Work out the finished part from the listing and answer in its coordinate system (mm). Face numbers are marked on the shaded views. A direction names the side the tool comes from. Coordinates: 2 decimals unless noted, no trailing zeros. Order: outer loops, then holes, each group sorted by start corner. A loop starts at its lowest first (then second) coordinate and runs counter-clockwise, first axis right, second up. Notation, with made-up numbers: (26, 84) -> (42, 84) arc R29 cw to (42, 117) -> close; hole circle Ø4 at (78.25, -1). An arc over 180 degrees is marked (long way). Write item = value, one per line. Start each with the question number.
Q1. For a pull along Z with two mould halves and no side action, classify the marked faces 5, 6 and 7 as +Z half, -Z half, draft (parallel to the pull), parting line (faces both ways), or undercut.
Q2. Which of the six approach directions +Z, -Z, +X, -X, +Y, -Y give full straight-line access (tool end or side, diameter ignored) to the marked faces 1, 2, 3 and 4?
Q3. Flat-ended cylindrical pins translate along their axes: pin 1 (2 mm diameter, centred on y = 60, z = -5, fed in from -X); pin 2 (1.3 mm diameter, centred on y = 59.5, z = -5, fed in from +X); pin 3 (1 mm diameter, centred on y = 13, z = 23, fed in from +X). Find the tip coordinate at first contact, or state that the pin passes through.
Q4. The part is cut by section B-B, the plane x = 0. Determine the outline of the cut face in (y, z), plus the area to 3 significant figures.
Q5. The part is cut by section A-A, the plane z = 0. Determine the outline of the cut face in (x, y).
Q6. Straight lines are drawn through the part: L1, parallel to Z at x = 0, y = 2.5; L2, parallel to Y at x = 10.8, z = 5; L3, parallel to Z at x = 10, y = 60. For each, find the intervals that lie inside material, in ascending order. Write a range as from..to.
Q7. The part is cut by section C-C, the plane y = 29. Determine the outline of the cut face in (x, z).
Q8. The part is cut by section D-D, the plane y = 50. Determine the outline of the cut face in (x, z), plus the area to 3 significant figures.
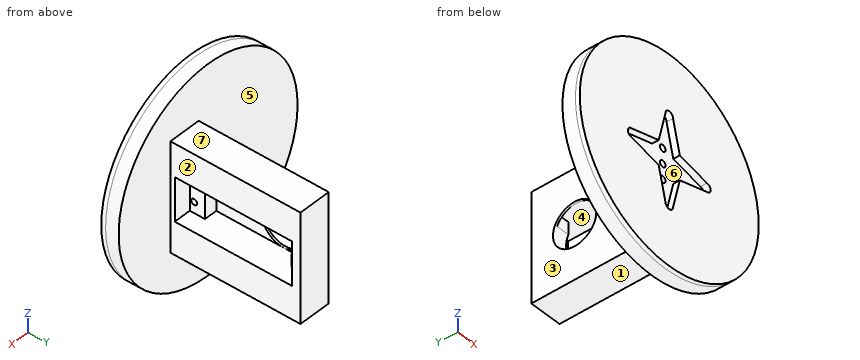
Autodesk Inventor part; units mm, degrees
ref_plane "YZ Plane" through (0, 0, 0) normal (1, 0, 0) x (0, 1, 0)
ref_plane "XZ Plane" through (0, 0, 0) normal (0, 1, 0) x (-1, 0, 0)
ref_plane "XY Plane" through (0, 0, 0) normal (0, 0, 1) x (1, 0, 0)
sketch "Sketch1" plane through (0, 0, 0) normal (0, 1, 0) x (-1, 0, 0)
  circle A0 centre (0, 0) radius 47.5
  dimension "d0" = 95
extrude "Extrusion1" add sketch "Sketch1" along normal blind 6
sketch "Sketch2" plane through (0, 6, 0) normal (0, 1, 0) x (1, 0, 0)
  circle A0 centre (0, 0) radius 7
  circle A1 centre (0, -7) radius 1.5
  circle A2 centre (0, 7) radius 1.5
  dimension "d3" = 14
  dimension "d4" = 3
  dimension "d5" = 3
extrude "Extrusion2" cut sketch "Sketch2" against normal blind 6 contours A2 A0 | A0 A2 | A1 A0 | A0 A1
sketch "Sketch3" plane through (0, 6, 0) normal (0, 1, 0) x (1, 0, 0)
  line L0 (0, 0) -> (5, 0)
  line L1 (5, 0) -> (5, -10)
  line L2 (5, -10) -> (0, -10)
  line L3 (0, -10) -> (0, 0)
  line L4 (5, 0) -> (0, 0)
  line L5 (0, 0) -> (0, 10)
  line L6 (0, 10) -> (5, 10)
  line L7 (5, 10) -> (5, 0)
  line L8 (5, 0) -> (20, 0)
  line L9 (20, 0) -> (20, -25)
  line L10 (20, -25) -> (5, -25)
  line L11 (5, -25) -> (5, 0)
  line L12 (20, 0) -> (5, 0)
  line L13 (5, 0) -> (5, 25)
  line L14 (5, 25) -> (20, 25)
  line L15 (20, 25) -> (20, 0)
  dimension "d8" = 5
  dimension "d9" = 10
  dimension "d10" = 10
  dimension "d11" = 15
  dimension "d12" = 25
  dimension "d13" = 25
extrude "Extrusion3" add sketch "Sketch3" along normal blind 60 contours L8 L9 L10 L11 L1 | L7 L13 L14 L15 L8
sketch "Sketch4" plane through (5, 6, -25) normal (-1, 0, 0) x (0, 0, 1)
  line L0 (50, 0) -> (50, 60)
  line L1 (50, 0) -> (48, 0)
  line L2 (48, 0) -> (48, 40)
  line L3 (48, 40) -> (50, 40)
  line L4 (50, 40) -> (50, 0)
  circle A0 centre (25, 40) radius 10
  point P0 (25, -6)
  dimension "d16" = 2
  dimension "d17" = 40
  dimension "d18" = 20
extrude "Extrusion4" cut sketch "Sketch4" against normal blind 20 contours A0
sketch "Sketch5" plane through (20, 6, 25) normal (1, 0, 0) x (0, 0, -1)
  circle A0 centre (25, 40) radius 10
  line L0 (25, 40) -> (30, 40)
  line L1 (30, 40) -> (30, 4)
  line L2 (30, 4) -> (25, 4)
  line L3 (25, 4) -> (25, 40)
  line L4 (25, 40) -> (20, 40)
  line L5 (20, 40) -> (20, 4)
  line L6 (20, 4) -> (25, 4)
  line L7 (25, 4) -> (25, 40)
  circle A1 centre (20, 4) radius 1.35
  circle A2 centre (30, 4) radius 1.35
  point P0 (25, -6)
  dimension "d21" = 5
  dimension "d22" = 36
  dimension "d23" = 5
  dimension "d24" = 36
  dimension "d25" = 2.7
  dimension "d26" = 2.7
extrude "Extrusion5" cut sketch "Sketch5" against normal blind 20 contours A1 L6 L5 | L5 L6 A1 | A2 L2 L1 | L1 L2 A2
sketch "Sketch6" plane through (20, 6, 25) normal (1, 0, 0) x (0, 0, -1)
  line L0 (25, 40) -> (30, 40)
  line L1 (30, 40) -> (30, 54)
  line L2 (30, 54) -> (25, 54)
  line L3 (25, 54) -> (25, 40)
  line L4 (25, 40) -> (20, 40)
  line L5 (20, 40) -> (20, 54)
  line L6 (20, 54) -> (25, 54)
  line L7 (25, 54) -> (25, 40)
  circle A0 centre (20, 54) radius 1.35
  circle A1 centre (30, 54) radius 1.35
  point P0 (25, -6)
  dimension "d29" = 5
  dimension "d30" = 14
  dimension "d31" = 5
  dimension "d32" = 14
  dimension "d33" = 2.7
  dimension "d34" = 2.7
extrude "Extrusion6" cut sketch "Sketch6" against normal blind 20 contours A1 L2 L1 | L1 L2 A1 | A0 L5 L6 | L6 L5 A0
sketch "Sketch7" plane through (20, 6, 25) normal (1, 0, 0) x (0, 0, -1)
  line L0 (20, 54) -> (30, 54)
  line L1 (30, 54) -> (30, 4)
  line L2 (30, 4) -> (20, 4)
  line L3 (20, 4) -> (20, 54)
  circle A0 centre (20, 54) radius 1.35
  line L4 (0, 0) -> (0, 60)
  line L5 (20, 54) -> (0, 54)
  line L6 (0, 54) -> (0, 49)
  line L7 (0, 49) -> (20, 49)
  line L8 (20, 49) -> (20, 54)
  circle A1 centre (25, 40) radius 10
  line L9 (25, 40) -> (15, 40)
  line L10 (15, 40) -> (15, 30)
  line L11 (15, 30) -> (25, 30)
  line L12 (25, 30) -> (25, 40)
  line L13 (25, 40) -> (35, 40)
  line L14 (35, 40) -> (35, 30)
  line L15 (35, 30) -> (25, 30)
  line L16 (25, 30) -> (25, 40)
  line L17 (35, 40) -> (15, 40)
  line L18 (15, 40) -> (15, 9)
  line L19 (15, 9) -> (35, 9)
  line L20 (35, 9) -> (35, 40)
  line L21 (15, 9) -> (35, 9)
  line L22 (35, 9) -> (35, 49)
  line L23 (35, 49) -> (15, 49)
  line L24 (15, 49) -> (15, 9)
  point P0 (25, -6)
  point P1 (30, 49)
  point P2 (30, 48.6603)
  point P3 (15, 49)
  point P4 (20, 48.6603)
  dimension "d37" = 10
  dimension "d38" = 50
  dimension "d39" = 5
  dimension "d40" = 10
  dimension "d41" = 10
  dimension "d42" = 10
  dimension "d43" = 31
  dimension "d44" = 40
extrude "Extrusion7" cut sketch "Sketch7" against normal blind 14 contours L3 A1 L24 L7 | L23 L22 A1 L1 | A1 L3 L11 L10 | L14 L15 L1 A1 | A1 L11 L3 | L11 L3 L19 L18 | L1 L15 A1 | L20 L19 L1 L15 | L11 L15 L1 L19 L3
sketch "Sketch8" plane through (20, 6, 25) normal (1, 0, 0) x (0, 0, -1)
  line L0 (15, 40) -> (15, 49)
  line L1 (15, 49) -> (35, 49)
  line L2 (35, 49) -> (35, 56)
  line L3 (35, 56) -> (15, 56)
  line L4 (15, 56) -> (15, 49)
  line L5 (35, 9) -> (15, 9)
  line L6 (15, 9) -> (35, 9)
  line L7 (35, 9) -> (35, 2)
  line L8 (35, 2) -> (15, 2)
  line L9 (15, 2) -> (15, 9)
  point P0 (25, -6)
  dimension "d47" = 20
  dimension "d48" = 7
  dimension "d49" = 20
  dimension "d50" = 7
sketch "Sketch9" plane through (20, 6, 25) normal (1, 0, 0) x (0, 0, -1)
  line L0 (15, 40) -> (15, 49)
  circle A0 centre (25, 40) radius 10
  line L1 (15, 49) -> (35, 49)
  line L2 (35, 49) -> (35, 40)
  line L3 (35, 40) -> (15, 40)
  line L4 (15, 40) -> (15, 49)
  line L5 (15, 49) -> (20, 49)
  line L6 (20, 49) -> (20.777, 49)
  line L7 (20.777, 49) -> (20.777, 48.469)
  line L8 (20.777, 48.469) -> (20, 48.469)
  line L9 (20, 48.469) -> (20, 49)
  line L10 (30, 49) -> (35, 49)
  line L11 (30, 49) -> (29.2041, 49)
  line L12 (29.2041, 49) -> (29.2041, 48.469)
  line L13 (29.2041, 48.469) -> (30, 48.469)
  line L14 (30, 48.469) -> (30, 49)
  line L15 (35, 49) -> (35, 9)
  line L16 (15, 56) -> (35, 56)
  line L17 (35, 56) -> (35, 49)
  line L18 (35, 49) -> (15, 49)
  line L19 (15, 49) -> (15, 56)
  line L20 (15, 9) -> (15, 49)
  line L21 (15, 9) -> (35, 9)
  line L22 (35, 9) -> (35, 2)
  line L23 (35, 2) -> (15, 2)
  line L24 (15, 2) -> (15, 9)
  point P0 (25, -6)
  point P1 (20, 48.6603)
  point P2 (30, 48.6603)
  dimension "d51" = 7
extrude "Extrusion8" cut sketch "Sketch9" against normal blind 12 contours L19 L16 L17 L1 A0 | L9 L1 A0 | L21 L22 L23 L24 | A0 L1 L14
sketch "Sketch10" plane through (8, 60, -5) normal (1, 0, 0) x (0, 0, -1)
  line L0 (-10, -5) -> (-10, -5.3397)
  line L1 (-10, -5) -> (0, -5)
  line L2 (0, -5) -> (0, -5.5581)
  line L3 (0, -5.5581) -> (-10, -5.5581)
  line L4 (-10, -5.5581) -> (-10, -5)
  point P0 (-5, -60)
extrude "Extrusion9" cut sketch "Sketch10" against normal blind 2
sketch "Sketch11" plane through (5, 6, -25) normal (-1, 0, 0) x (0, 0, 1)
  point P0 (25, -6)
sketch "Sketch12" plane through (0, 0, 0) normal (0, -1, 0) x (1, 0, 0)
  circle A0 centre (0, 0) radius 1.5
  dimension "d56" = 3
extrude "Extrusion10" cut sketch "Sketch12" against normal blind 13.8125
sketch "Sketch13" plane through (0, 0, 0) normal (0, -1, 0) x (1, 0, 0)
  circle A0 centre (0, 0) radius 1.5
  circle A1 centre (0, 0) radius 47.5
  circle A2 centre (0, 7) radius 1.5
  circle A3 centre (0, 7) radius 1.5
  circle A4 centre (0, 0) radius 1.5
  circle A5 centre (0, -7) radius 1.5
  circle A6 centre (0, -7) radius 1.5
  dimension "d59" = 3
extrude "Extrusion11" add sketch "Sketch13" along normal blind 2
sketch "Sketch14" plane through (0, -2, 0) normal (0, -1, 0) x (1, 0, 0)
  circle A0 centre (0, 0) radius 1.5
  circle A1 centre (0, 0) radius 7
  line L0 (0, 0) -> (0, -20)
  line L1 (0, -20) -> (0, 20)
  line L2 (0, 0) -> (20, 0)
  line L3 (20, 0) -> (-20, 0)
  circle A2 centre (0, 20) radius 2
  circle A3 centre (-20, 0) radius 2
  circle A4 centre (0, -20) radius 2
  circle A5 centre (20, 0) radius 2
  line L4 (2, 20) -> (7, 0)
  line L5 (-2, 20) -> (-7, 0)
  line L6 (20, 25) -> (20, -25)
  circle A6 centre (0, 7) radius 1.5
  line L7 (20, 2) -> (0, 7)
  circle A7 centre (0, -7) radius 1.5
  line L8 (20, -2) -> (0, -7)
  line L9 (2, -20) -> (7, 0)
  line L10 (-2, -20) -> (-7, 0)
  line L11 (-20, 2) -> (0, 7)
  line L12 (-20, -2) -> (0, -7)
  point P0 (6.1765, 3.2941)
  point P1 (6.1765, -3.2941)
  point P2 (-6.1765, -3.2941)
  point P3 (3.2941, -6.1765)
  point P4 (1.4914, -6.8393)
  point P5 (-1.4914, -6.8393)
  point P6 (-3.2941, -6.1765)
  point P7 (-1.4552, -6.6362)
  point P8 (1.4552, -6.6362)
  point P9 (3.2941, 6.1765)
  point P10 (1.4552, 6.6362)
  point P11 (-1.4552, 6.6362)
  point P12 (-3.2941, 6.1765)
  point P13 (-1.4914, 6.8393)
  point P14 (1.4914, 6.8393)
  point P15 (5.6, 5.6)
  point P16 (-5.6, 5.6)
  point P17 (-5.6, -5.6)
  point P18 (5.6, -5.6)
  dimension "d62" = 14
  dimension "d63" = 20
  dimension "d64" = 40
  dimension "d65" = 20
  dimension "d66" = 40
  dimension "d67" = 4
  dimension "d68" = 4
  dimension "d69" = 4
  dimension "d70" = 4
extrude "Extrusion12" cut sketch "Sketch14" against normal blind 3 contours L2 L9 A1 L8 A7 L0 A0 | A0 L1 A6 L7 A1 L4 L2 | A0 L3 L5 A1 L11 A6 L1 | L0 A7 L12 A1 L10 L3 A0 | L2 A5 L8 L9 A1 | A1 L4 L7 A5 L2 | A1 L7 L4 | L9 L8 A1 | A5 L6 L2 | L2 L6 A5 | L3 A3 L11 L5 A1 | A1 L10 L12 A3 L3 | A1 L5 | A1 A6 L1 A2 L4 L7 | L8 L9 A4 L0 A7 A1 | L6 A5 | L5 L11 A1 | A1 L12 L10 | A3 | A1 L11 L5 A2 L1 A6 | A7 L0 A4 L10 L12 A1 | A2 | A4
sketch "Sketch16" plane through (0, -2, 0) normal (0, -1, 0) x (1, 0, 0)
  line L0 (-8.315, -3.9346) -> (-4.5008, -3.9346)
  line L1 (-4.5008, -3.9346) -> (-4.5008, 0)
  line L2 (-4.5008, 0) -> (-8.315, 0)
  line L3 (-8.315, 0) -> (-8.315, -3.9346)
  line L4 (-3.8, -5.15) -> (4.3559, -5.15)
  line L5 (4.3559, -5.15) -> (4.3559, -8.3953)
  line L6 (4.3559, -8.3953) -> (-3.8, -8.3953)
  line L7 (-3.8, -8.3953) -> (-3.8, -5.15)
  line L8 (-3.8, 4.0171) -> (3.8, 4.0171)
  line L9 (3.8, 4.0171) -> (3.8, 8.6071)
  line L10 (3.8, 8.6071) -> (-3.8, 8.6071)
  line L11 (-3.8, 8.6071) -> (-3.8, 4.0171)
  line L12 (6, -4.3589) -> (8, -4.3589)
  line L13 (5.3903, 4.0171) -> (8, 4.0171)
  line L14 (8, 4.0171) -> (8, -4.3589)
  line L15 (8, -4.3589) -> (5.3903, -4.3589)
  line L16 (5.3903, -4.3589) -> (5.3903, 4.0171)
  point P0 (0, 0)
extrude "Extrusion13" cut sketch "Sketch16" against normal blind 3
sketch "Sketch17" plane through (8, 6, 25) normal (1, 0, 0) x (0, 0, -1)
  point P0 (25, -6)
sketch "Sketch18" plane through (6, 15, 10) normal (0, 0, -1) x (-1, 0, 0)
  point P0 (6, -15)
sketch "Sketch19" plane through (6, 15, 10) normal (0, 1, 0) x (1, 0, 0)
  point P0 (-6, 10)
sketch "Sketch20" plane through (8, 6, 25) normal (1, 0, 0) x (0, 0, -1)
  line L0 (35, 56) -> (35, 2)
  line L1 (15, 49) -> (20.6411, 49)
  line L2 (35, 56) -> (15, 56)
  line L3 (15, 56) -> (15, 49)
  line L4 (15, 49) -> (35, 49)
  line L5 (35, 49) -> (35, 56)
  circle A0 centre (25, 40) radius 10
  circle A1 centre (25, 40) radius 10
  line L6 (35, 40) -> (35, 9)
  line L7 (35, 2) -> (15, 2)
  line L8 (35, 9) -> (15, 9)
  line L9 (15, 9) -> (15, 2)
  line L10 (15, 2) -> (35, 2)
  line L11 (35, 2) -> (35, 9)
  circle A2 centre (20, 54) radius 1.35
  circle A3 centre (20, 54) radius 0.875
  circle A4 centre (30, 54) radius 1.35
  circle A5 centre (30, 54) radius 0.875
  circle A6 centre (30, 4) radius 1.35
  circle A7 centre (30, 4) radius 0.875
  circle A8 centre (20, 4) radius 1.35
  circle A9 centre (20, 4) radius 0.875
  point P0 (25, -6)
  point P1 (29.3589, 49)
extrude "Extrusion14" add sketch "Sketch20" along normal blind 8 contours L0 L7 L9 L8 | L0 L4 A0 L1 L3 L2
sketch "Sketch21" plane through (5, 6, -25) normal (-1, 0, 0) x (0, 0, 1)
  circle A0 centre (30, 54) radius 1.35
  circle A1 centre (30, 54) radius 1.35
  circle A2 centre (20, 54) radius 1.35
  circle A3 centre (20, 54) radius 1.35
  circle A4 centre (30, 4) radius 1.35
  circle A5 centre (30, 4) radius 1.35
  circle A6 centre (20, 4) radius 1.35
  circle A7 centre (20, 4) radius 1.35
  point P0 (25, -6)
extrude "Extrusion15" add sketch "Sketch21" against normal blind 2
sketch "Sketch22" plane through (16, 6, 25) normal (1, 0, 0) x (0, 0, -1)
  line L0 (15, 56) -> (35, 56)
  line L1 (15, 49) -> (15, 56)
  line L2 (35, 56) -> (15, 56)
  line L3 (15, 56) -> (15, 49)
  line L4 (15, 49) -> (35, 49)
  line L5 (35, 49) -> (35, 56)
  arc A0 (35, 40) -> (29.3589, 49) centre (25, 40) ccw
  circle A1 centre (25, 40) radius 10
  line L6 (35, 9) -> (15, 9)
  line L7 (35, 2) -> (15, 2)
  line L8 (15, 9) -> (35, 9)
  line L9 (35, 9) -> (35, 2)
  line L10 (35, 2) -> (15, 2)
  line L11 (15, 2) -> (15, 9)
  circle A2 centre (30, 54) radius 1.35
  circle A3 centre (30, 54) radius 1.35
  circle A4 centre (20, 54) radius 1.35
  circle A5 centre (20, 54) radius 1.35
  circle A6 centre (30, 4) radius 1.35
  circle A7 centre (30, 4) radius 1.35
  circle A8 centre (20, 4) radius 1.35
  circle A9 centre (20, 4) radius 1.35
  point P0 (25, -6)
  point P1 (20.6411, 49)
extrude "Extrusion16" cut sketch "Sketch22" against normal blind 4 contours L0 L5 L4 A1 L1 | L9 L7 L11 L6
properties part number "FinalNewbaseTop"
Model answer:
q1.face_5 = draft
q1.face_6 = undercut
q1.face_7 = +Z half
q2.face_1 = -Z, +X, -X, +Y
q2.face_2 = +Z, -Z, +X, +Y
q2.face_3 = +Z, -Z, -X, +Y
q2.face_4 = +X
q3.pin_1 = 5
q3.pin_2 = 7
q3.pin_3 = 20
q4.outline = (-2, -47.5) -> (6, -47.5) -> (6, -8.5) -> (1, -8.5) -> (1, -22) -> (-2, -22) -> close; (-2, 22) -> (1, 22) -> (1, 8.5) -> (6, 8.5) -> (6, 47.5) -> (-2, 47.5) -> close; (1, -5.5) -> (6, -5.5) -> (6, -1.5) -> (1, -1.5) -> close; (1, 1.5) -> (6, 1.5) -> (6, 5.5) -> (1, 5.5) -> close
q4.area = 583 mm2
q5.outline = (-47.5, -2) -> (-22, -2) -> (-22, 1) -> (-1.5, 1) -> (-1.5, 6) -> (-47.5, 6) -> close; (1.5, 1) -> (22, 1) -> (22, -2) -> (47.5, -2) -> (47.5, 6) -> (20, 6) -> (20, 8) -> (12, 8) -> (12, 15) -> (6, 15) -> (6, 36) -> (5, 36) -> (5, 6) -> (1.5, 6) -> close; (5, 56) -> (12, 56) -> (12, 62) -> (20, 62) -> (20, 66) -> (5, 66) -> close
q6.L1 = -47.5..-8.5, -5.5..-1.5, 1.5..5.5, 8.5..47.5
q6.L2 = -2..8.65, 11.35..15, 55..58.65, 61.35..66
q6.L3 = -25..-6.35, -3.65..3.65, 6.35..25
q7.outline = (5, -25) -> (20, -25) -> (20, -10) -> (6, -10) -> (6, 10) -> (20, 10) -> (20, 25) -> (5, 25) -> close
q8.outline = (5, -25) -> (20, -25) -> (20, -10) -> (6, -10) -> (6, -9.17) -> (5, -9.17) -> close; (5, 9.17) -> (6, 9.17) -> (6, 10) -> (20, 10) -> (20, 25) -> (5, 25) -> close
q8.area = 452 mm2
